```python
from build123d import *

# Parameters (mm, degrees)
F1_DEPTH = 101.6


with BuildPart() as f1:
    # F0 (on Front) → F1 (new body)
    with BuildSketch(Plane.XZ):
        with BuildLine():
            ThreePointArc((-20.63977, -29.72378), (-32.065525, -16.772159), (-36.187058, 0))
            Line((-36.187058, 0), (-36.187058, 27.704396))
            ThreePointArc((-36.187058, 27.704396), (-38.341088, 30.969492), (-41.983402, 32.395763))
            Line((-41.983402, 32.395763), (-50.8, 32.395763))
            Line((-50.8, 32.395763), (-50.8, 0))
            ThreePointArc((-50.8, 0), (-44.088108, -25.236456), (-25.726035, -43.804237))
            Line((-25.726035, -43.804237), (0, -43.804237))
            Line((0, -43.804237), (25.726035, -43.804237))
            ThreePointArc((25.726035, -43.804237), (44.088108, -25.236456), (50.8, 0))
            Line((50.8, 0), (50.8, 32.395763))
            Line((50.8, 32.395763), (41.983402, 32.395763))
            ThreePointArc((41.983402, 32.395763), (38.341088, 30.969492), (36.187058, 27.704396))
            Line((36.187058, 27.704396), (36.187058, 0))
            ThreePointArc((36.187058, 0), (32.065525, -16.772159), (20.63977, -29.72378))
            ThreePointArc((20.63977, -29.72378), (16.846551, -31.580554), (12.671795, -32.218926))
            Line((12.671795, -32.218926), (0, -32.218926))
            Line((0, -32.218926), (-12.671795, -32.218926))
            ThreePointArc((-12.671795, -32.218926), (-16.846551, -31.580554), (-20.63977, -29.72378))
        make_face()
    extrude(amount=F1_DEPTH)


solid = f1.part
```
Model file for the job. Use its own axes, mm. A direction names the side the tool comes from. Coordinates: 2 decimals unless noted, no trailing zeros. Loops run counter-clockwise (first coordinate to the right, second up) from the corner with the lowest first, then second, coordinate; pieces in that order, holes last. Notation, with made-up numbers: (42.5, -20.75) - (94.5, -20.75) arc R12 ccw to (94.5, -6.75) - close; hole circle Ø1 at (70, 19). An arc over 180 degrees is marked (long way). Write item = value, one per line. Start each with the question number.
Item 1: Pull direction X, two halves, no side cores. Call faces 3 (the face through (0, -50, -32.219)), 4 (the face through (-46, -50, 32.396)), 5 (the face through (43.9, -50.09, -25.56)): +X half, -X half, draft (parallel to the pull), parting line (faces both ways), or undercut.
Item 2: Drop flat-ended pins along their axis: pin 1 Ø6 at (y, z) = (-85, -15) entering from -X; pin 2 Ø1.5 at (y, z) = (-27.5, -25) entering from +X; pin 3 Ø5 at (x, y) = (-14.5, -33.5) entering from +Z. Give the stop position or say it passes through.
Item 3: Saw through at B-B, the plane y = -52.5. List the corners of the cut face in (x, z).
Item 4: 3-axis set-ups, long thin cutter, end or side, ignore diameter. For faces 1 (the face through (0, -50, -43.804)), 2 (the face through (32.178, -50.089, -16.555)): which of +Z, -Z, +X, -X, +Y, -Y reach the whole face in a straight line?
Item 5: Saw through at D-D, the plane x = -43.5. List the corners of the cut face in (y, z), then the cut area to 3 significant figures.
Item 6: Wall check: probe 1 along X at (y, z) = (-74.5, 5); probe 2 along Z at (x, y) = (2, -77); probe 3 along X at (y, z) = (-12, -6). Give the ranges that are in metal, low to high. Write a range as [from, to].
Item 7: Saw through at C-C, the plane z = -24.5. List the corners of the cut face in (x, y), then the cut area to 3 significant figures.
Item 8: Saw through at A-A, the plane z = 4. List the corners of the cut face in (x, y).
Answers:
q1.face_3 = undercut
q1.face_4 = draft
q1.face_5 = +X half
q2.pin_1 = -49.36
q2.pin_2 = 44.64
q2.pin_3 = -31.53
q3.outline = (-50.8, 0) arc R50.8 ccw to (-25.73, -43.8) - (25.73, -43.8) arc R50.8 ccw to (50.8, 0) - (50.8, 32.4) - (41.98, 32.4) arc R6.47 ccw to (36.19, 27.7) - (36.19, 0) arc R36.19 cw to (20.64, -29.72) arc R13.97 cw to (12.67, -32.22) - (-12.67, -32.22) arc R13.97 cw to (-20.64, -29.72) arc R36.19 cw to (-36.19, 0) - (-36.19, 27.7) arc R6.47 ccw to (-41.98, 32.4) - (-50.8, 32.4) - close
q4.face_1 = -Z, +X, -X, +Y, -Y
q4.face_2 = +Z, +Y, -Y
q5.outline = (-101.6, -26.24) - (0, -26.24) - (0, 32.4) - (-101.6, 32.4) - close
q5.area = 5,960 mm2
q6.probe_1 = [-50.8, -36.19], [36.19, 50.8]
q6.probe_2 = [-43.8, -32.22]
q6.probe_3 = [-50.44, -35.69], [35.69, 50.44]
q7.outline = (-44.5, -101.6) - (-26.63, -101.6) - (-26.63, 0) - (-44.5, 0) - close; (26.63, -101.6) - (44.5, -101.6) - (44.5, 0) - (26.63, 0) - close
q7.area = 3,630 mm2
q8.outline = (-50.8, -101.6) - (-36.19, -101.6) - (-36.19, 0) - (-50.8, 0) - close; (36.19, -101.6) - (50.8, -101.6) - (50.8, 0) - (36.19, 0) - close
